Verification items for the finished model (mm, model axes). Face numbers are marked on the shaded views. A direction names the side the tool comes from. Coordinates: 2 decimals unless noted, no trailing zeros. Order: outer loops, then holes, each group sorted by start corner. A loop starts at its lowest first (then second) coordinate and runs counter-clockwise, first axis right, second up. Notation, with made-up numbers: (22.5, 54) -> (29.5, 54) arc R23 cw to (29.5, 75) -> close; hole circle Ø3 at (46, 67). An arc over 180 degrees is marked (long way). Write item = value, one per line. Start each with the question number.
1. Release check for a two-part mould opening along Z. For the marked faces 1, 2 and 3 record: +Z half, -Z half, draft (parallel to the pull), parting line (faces both ways), or undercut.
2. Thickness scan on line 1 along Y through (x, z) = (0, 41.25); line 2 along Z through (x, y) = (-93.5, -27); line 3 along Y through (x, z) = (19, 47.5). Record the ranges inside material, lowest first. Write a range as from..to.
3. Cross-section at D-D on y = 46.5. Record the cut outline in (x, z).
4. Go/stop test with flat-tipped pins: P1, Ø5, axis at x = -78.5, z = 32, coming from the -Y side; P2, Ø8, axis at x = 102.5, z = 20.5, coming from the -Y side; P3, Ø3, axis at x = 56.5, z = 32.5, coming from the +Y side. Record where each tip stops, or that it passes through.
5. Set-up check for the marked faces 4, 5, 6, 7 and 8: record each of +Z, -Z, +X, -X, +Y, -Y from which the full face is reachable in a straight line by a thin tool's end or side.
6. Cross-section at A-A on y = 87.5. Record the cut outline in (x, z).
7. Cross-section at C-C on z = 2.5. Record the cut outline in (x, y), plus the area to 3 significant figures.
8. Cross-section at B-B on x = 5.5. Record the cut outline in (y, z).
from build123d import *

# Parameters (mm, degrees)
F1_DEPTH  = 50
F2_W      = 25
F2_H      = 25
F3_DEPTH  = 15
F4_W      = 25
F4_H      = 25
F5_DEPTH  = 15
F6_W      = 25
F6_H      = 25
F7_DEPTH  = 15
F8_W      = 25
F8_H      = 25
F9_DEPTH  = 15
F11_DEPTH = 5
F13_DEPTH = 5
F15_DEPTH = 5
F17_DEPTH = 5
F18_R     = 100
F19_DEPTH = 25
F20_R     = 100
F21_DEPTH = 20


with BuildPart() as f1:
    # F0 (on Top) → F1 (new body)
    with BuildSketch(Plane.XY):
        Polygon((-92.3879532511, -92.3879532511), (0, -130.6562964876), (92.3879532511, -92.3879532511), (130.6562964876, 0), (92.3879532511, 92.3879532511), (0, 130.6562964876), (-92.3879532511, 92.3879532511), (-130.6562964876, 0), align=None)
    extrude(amount=F1_DEPTH)

    # F2 (on face) → F3 (cut)
    with BuildSketch(Plane(origin=(-46.1939766256, -111.5221248694, 0), x_dir=(0.9238795325, -0.3826834324, 0), z_dir=(-0.3826834324, -0.9238795325, 0))):
        with Locations((0, 25)):
            Rectangle(F2_W, F2_H)
    extrude(amount=-F3_DEPTH, mode=Mode.SUBTRACT)

    # F4 (on face) → F5 (cut)
    with BuildSketch(Plane(origin=(-111.5221248694, 46.1939766256, 0), x_dir=(-0.3826834324, -0.9238795325, 0), z_dir=(-0.9238795325, 0.3826834324, 0))):
        with Locations((0, 25)):
            Rectangle(F4_W, F4_H)
    extrude(amount=-F5_DEPTH, mode=Mode.SUBTRACT)

    # F6 (on face) → F7 (cut)
    with BuildSketch(Plane(origin=(46.1939766256, 111.5221248694, 0), x_dir=(-0.9238795325, 0.3826834324, 0), z_dir=(0.3826834324, 0.9238795325, 0))):
        with Locations((0, 25)):
            Rectangle(F6_W, F6_H)
    extrude(amount=-F7_DEPTH, mode=Mode.SUBTRACT)

    # F8 (on face) → F9 (cut)
    with BuildSketch(Plane(origin=(111.5221248694, -46.1939766256, 0), x_dir=(0.3826834324, 0.9238795325, 0), z_dir=(0.9238795325, -0.3826834324, 0))):
        with Locations((0, 25)):
            Rectangle(F8_W, F8_H)
    extrude(amount=-F9_DEPTH, mode=Mode.SUBTRACT)

    # F10 (on face) → F11 (cut)
    with BuildSketch(Plane(origin=(46.1939766256, -111.5221248694, 0), x_dir=(0.9238795325, 0.3826834324, 0), z_dir=(0.3826834324, -0.9238795325, 0))):
        Polygon((12.4999989995, 3.3493643278), (25, 24.9999988448), (12.5000010005, 46.650634517), (-12.4999989995, 46.6506356722), (-25, 25.0000011552), (-12.5000010005, 3.349365483), align=None)
    extrude(amount=-F11_DEPTH, mode=Mode.SUBTRACT)

    # F12 (on face) → F13 (cut)
    with BuildSketch(Plane(origin=(111.5221248694, 46.1939766256, 0), x_dir=(-0.3826834324, 0.9238795325, 0), z_dir=(0.9238795325, 0.3826834324, 0))):
        Polygon((12.4999987427, 3.3493641795), (25, 24.9999985481), (12.5000012573, 46.6506343687), (-12.4999987427, 46.6506358205), (-25, 25.0000014519), (-12.5000012573, 3.3493656313), align=None)
    extrude(amount=-F13_DEPTH, mode=Mode.SUBTRACT)

    # F14 (on face) → F15 (cut)
    with BuildSketch(Plane(origin=(-111.5221248694, -46.1939766256, 0), x_dir=(0.3826834324, -0.9238795325, 0), z_dir=(-0.9238795325, -0.3826834324, 0))):
        Polygon((12.5, 46.6506350946), (-12.5, 46.6506350946), (-25, 25), (-12.5, 3.3493649054), (12.5, 3.3493649054), (25, 25), align=None)
    extrude(amount=-F15_DEPTH, mode=Mode.SUBTRACT)

    # F16 (on face) → F17 (cut)
    with BuildSketch(Plane(origin=(-46.1939766256, 111.5221248694, 0), x_dir=(-0.9238795325, -0.3826834324, 0), z_dir=(-0.3826834324, 0.9238795325, 0))):
        Polygon((12.5, 46.6506350946), (-12.5, 46.6506350946), (-25, 25), (-12.5, 3.3493649054), (12.5, 3.3493649054), (25, 25), align=None)
    extrude(amount=-F17_DEPTH, mode=Mode.SUBTRACT)

    # F18 (on face) → F19 (cut)
    with BuildSketch(Plane.XY.offset(50)):
        Circle(F18_R)
    extrude(amount=-F19_DEPTH, mode=Mode.SUBTRACT)

    # F20 (on face) → F21 (join)
    with BuildSketch(Plane(origin=(0, 0, 0), x_dir=(1, 0, 0), z_dir=(0, 0, -1))):
        Circle(F20_R)
    extrude(amount=F21_DEPTH)


with BuildPart() as f1_1:
    # F22: moved
    add(f1.part.moved(Location((0, 0, 10))))


solid = f1_1.part
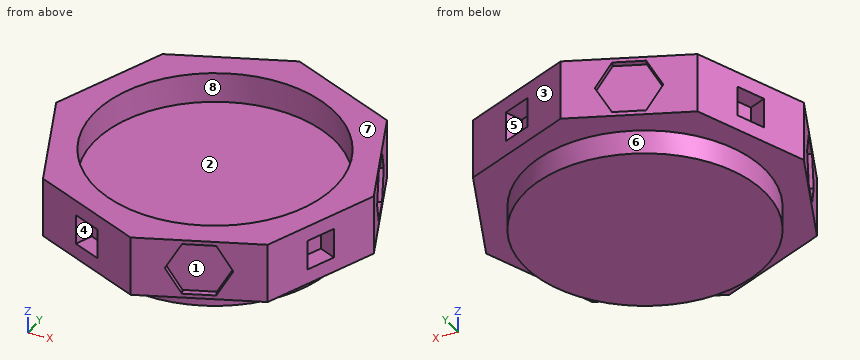
Worked out:
q1.face_1 = undercut
q1.face_2 = +Z half
q1.face_3 = draft
q2.line_1 = -130.66..-100, 100..130.66
q2.line_2 = -10..35
q2.line_3 = -122.79..-98.18, 98.18..122.79
q3.outline = (-111.4, 10) -> (-88.53, 10) -> (-88.53, -10) -> (88.53, -10) -> (88.53, 10) -> (111.4, 10) -> (111.4, 13.35) -> (105.98, 13.35) -> (105.98, 56.65) -> (111.4, 56.65) -> (111.4, 60) -> (88.53, 60) -> (88.53, 35) -> (-88.53, 35) -> (-88.53, 60) -> (-111.4, 60) -> (-111.4, 47.5) -> (-95.16, 47.5) -> (-95.16, 22.5) -> (-111.4, 22.5) -> close
q4.P1 = -99.18
q4.P2 = -77.63
q4.P3 = 106.74
q5.face_4 = -Y
q5.face_5 = +Y
q5.face_6 = -Z
q5.face_7 = +Z, +X, -X, +Y, -Y
q5.face_8 = +Z
q6.outline = (-94.41, 10) -> (-48.41, 10) -> (-48.41, -10) -> (48.41, -10) -> (48.41, 10) -> (94.41, 10) -> (94.41, 60) -> (48.41, 60) -> (48.41, 35) -> (-48.41, 35) -> (-48.41, 60) -> (-94.41, 60) -> close
q7.outline = circle Ø200 at (0, 0)
q7.area = 31,400 mm²
q8.outline = (-128.38, 10) -> (-99.85, 10) -> (-99.85, -10) -> (99.85, -10) -> (99.85, 10) -> (128.38, 10) -> (128.38, 60) -> (99.85, 60) -> (99.85, 35) -> (-99.85, 35) -> (-99.85, 60) -> (-128.38, 60) -> close
